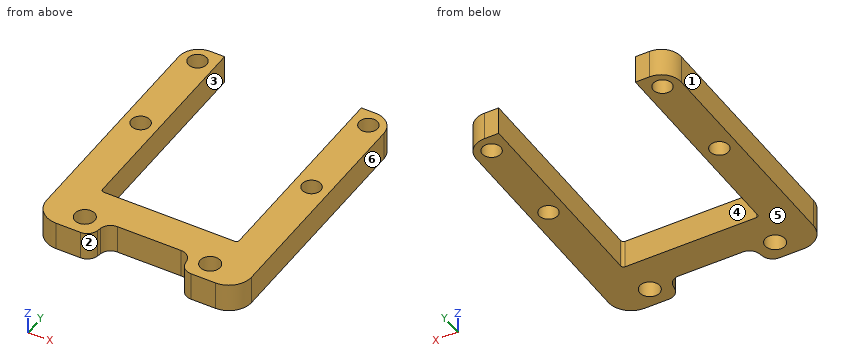
```python
from build123d import *

# Parameters (mm, degrees)
ESQUISSE1_R        = 3.25
ESQUISSE1_R_2      = 3.5
BOSS_EXTRU_1_DEPTH = 10
CONG_1_R           = 4
CONG_2_R           = 8
CONG_3_R           = 7
CONG_4_R           = 1


with BuildPart() as part:
    # Esquisse1 → Boss.-Extru.1 (new body)
    with BuildSketch(Plane.XY):
        Polygon((24, 110), (24, 36), (0, 36), (0, 24), (14.5, 24), (16.055042473, 16), (36, 16), (36, 110), align=None)
        with Locations((30, 104)):
            Circle(ESQUISSE1_R, mode=Mode.SUBTRACT)
        with Locations((22, 23)):
            Circle(ESQUISSE1_R_2, mode=Mode.SUBTRACT)
        with Locations((30, 70)):
            Circle(ESQUISSE1_R, mode=Mode.SUBTRACT)
    boss_extru_1 = extrude(amount=BOSS_EXTRU_1_DEPTH)

    # Symétrie2: Boss.-Extru.1 across plane
    add(boss_extru_1.mirror(Plane(origin=(0, 36, 10), x_dir=(0, 0, 1), z_dir=(1, 0, 0))))

    # Congé1
    cong_1_edges = [part.edges().sort_by_distance(p)[0] for p in [
        (16.055042473, 16, 5),
        (14.5, 24, 5),
        (-14.5, 24, 5),
        (-16.055042473, 16, 5),
    ]]
    fillet(cong_1_edges, radius=CONG_1_R)

    # Congé2
    cong_2_edges = [part.edges().sort_by_distance(p)[0] for p in [
        (36, 16, 5),
        (-36, 16, 5),
    ]]
    fillet(cong_2_edges, radius=CONG_2_R)

    # Congé3
    cong_3_edges = [part.edges().sort_by_distance(p)[0] for p in [
        (36, 110, 5),
        (-36, 110, 5),
    ]]
    fillet(cong_3_edges, radius=CONG_3_R)

    # Congé4
    cong_4_edges = [part.edges().sort_by_distance(p)[0] for p in [
        (24, 36, 5),
        (-24, 36, 5),
    ]]
    fillet(cong_4_edges, radius=CONG_4_R)


solid = part.part
```
Here's how the part is built. I have some questions about the finished solid (model axes, mm). Face numbers are marked on the shaded views. A direction names the side the tool comes from. Round coordinates to 2 decimals unless told otherwise and drop trailing zeros. Order: outer loops, then holes, each group sorted by start corner. A loop starts at its lowest first (then second) coordinate and runs counter-clockwise, first axis right, second up. Notation, with made-up numbers: M 0,50 L 47,50 A31 ccw 47,87 Z; hole C 1.5,8.25 d4. An arc over 180 degrees is marked long. Answer as CSV lines item,"result".
Item 1: Which directions (+Z, -Z, +X, -X, +Y, -Y) give clear straight access to the entire face, cutting with the end or side of a thin tool? Please do the marked faces 1, 2 and 3.
From the geometry:
face 1,"+Z, -Z, -X, +Y, -Y"
face 2,"+Z, -Z, -Y"
face 3,"+Z, -Z, +Y"
Item 2: For pin 1 (5 mm diameter, centred on x = -16.5, z = 1.5, fed in from +Y); pin 2 (5 mm diameter, centred on x = 4.5, z = 7, fed in from -Y), each with a flat end and sliding along its axis, tell me the tip position at first contact or that it passes through.
From the geometry:
pin 1,"y = 36"
pin 2,"y = 24"
Item 3: Imagine slicing it at D-D on y = 104. List the corners of the cut face in (x, z) for me, and give its area (3 significant figures).
From the geometry:
outline,"M -35.93,0 L -33.25,0 L -33.25,10 L -35.93,10 Z; M -26.75,0 L -24,0 L -24,10 L -26.75,10 Z; M 24,0 L 26.75,0 L 26.75,10 L 24,10 Z; M 33.25,0 L 35.93,0 L 35.93,10 L 33.25,10 Z"
area,"109 mm2"
Item 4: Imagine slicing it at B-B on x = 22. List the corners of the cut face in (y, z) for me, and give its area (3 significant figures).
From the geometry:
outline,"M 16,0 L 19.5,0 L 19.5,10 L 16,10 Z; M 26.5,0 L 36,0 L 36,10 L 26.5,10 Z"
area,"130 mm2"
Item 5: Imagine slicing it at A-A on z = 5.5. List the corners of the cut face in (x, y) for me, and give its area (3 significant figures).
From the geometry:
outline,"M -36,24 A8 ccw -28,16 L -19.35,16 A4 ccw -15.43,19.24 L -15.13,20.76 A4 cw -11.2,24 L 11.2,24 A4 cw 15.13,20.76 L 15.43,19.24 A4 ccw 19.35,16 L 28,16 A8 ccw 36,24 L 36,103 A7 ccw 29,110 L 24,110 L 24,37 A1 cw 23,36 L -23,36 A1 cw -24,37 L -24,110 L -29,110 A7 ccw -36,103 Z; hole C -30,70 d6.5; hole C -30,104 d6.5; hole C -22,23 d7; hole C 22,23 d7; hole C 30,70 d6.5; hole C 30,104 d6.5"
area,"2,710 mm2"
Item 6: We'd pull the mould along X, two halves only. Please class the marked faces 4, 5 and 6: +X half, -X half, draft (parallel to the pull), parting line (faces both ways), or undercut.
From the geometry:
face 4,"undercut"
face 5,"draft"
face 6,"+X half"
Item 7: Imagine slicing it at C-C on y = 47. List the corners of the cut face in (x, z) for me, and give its area (3 significant figures).
From the geometry:
outline,"M -36,0 L -24,0 L -24,10 L -36,10 Z; M 24,0 L 36,0 L 36,10 L 24,10 Z"
area,"240 mm2"
Item 8: Please list where these lines run through material, in increasing order: L1, parallel to Y at x = 22, z = 3.5; L2, parallel to X at y = 94.5, z = 6; L3, parallel to Y at x = -30, z = 4.75. Write a range as [from, to].
From the geometry:
L1,"[16, 19.5], [26.5, 36]"
L2,"[-36, -24], [24, 36]"
L3,"[16.25, 66.75], [73.25, 100.75], [107.25, 109.93]"
